Could you check a few things on this drawing? It's one solid part, dimensions in mm from its lowest x, y, z. A direction names the side the tool comes from. Round coordinates to 2 decimals unless told otherwise and drop trailing zeros. Loops run counter-clockwise (first coordinate to the right, second up) from the corner with the lowest first, then second, coordinate; pieces in that order, holes last. Notation, with made-up numbers: M 15.5,51 L 28.5,51 A17 cw 28.5,70 Z; hole C 7.5,-8 d10. An arc over 180 degrees is marked long. Put each result on its own line as item: value. Start each with the question number.
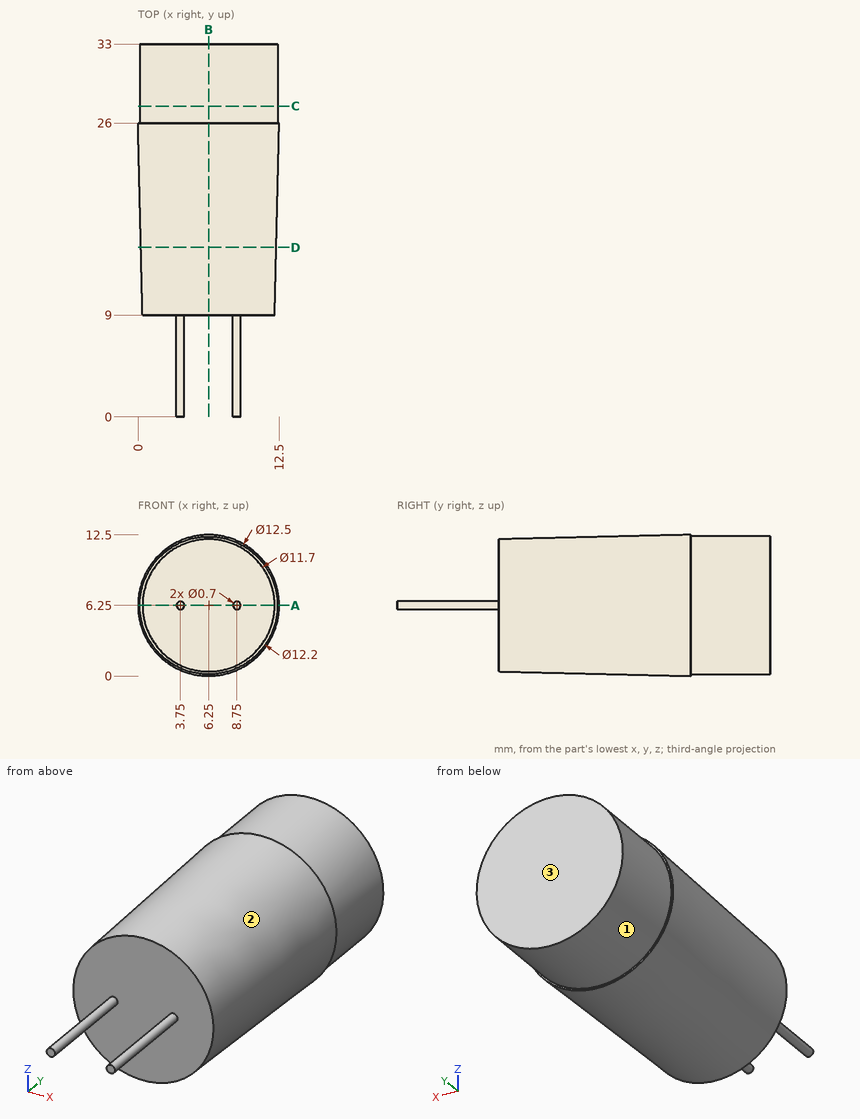
1) Suppose I cut it at B-B (x = 6.25). Write out the boundary of the cut face in (y, z).
2) I'm going to push flat-ended pins straight in: P1, Ø5, axis at y = 21, z = 1.5, coming from the -X side; P2, Ø3, axis at y = 7, z = 7.5, coming from the +X side; P3, Ø4, axis at x = 5, y = 23, coming from the -Z side. Where does each tip first touch, or does it pass through?
3) Suppose I cut it at D-D (y = 15). Write out the boundary of the cut face in (x, z), plus the area to 3 significant figures.
4) If I drill on probe 1 along Y at (x, z) = (2.75, 2.75); probe 2 along X at (y, z) = (28, 6.25); probe 3 along X at (y, z) = (4.5, 6), over which ranges is the centre line in solid material (lowest first)? Write a range as from..to.
5) Suppose I cut it at A-A (z = 6.25). Write out the boundary of the cut face in (x, y), plus the area to 3 significant figures.
6) On a 3-axis mill with a long thin cutter (end or side, diameter ignored), from which of +Z, -Z, +X, -X, +Y, -Y can I reach the whole of each face in a straight line? I mean the marked faces 1, 2 and 3. Say none if no direction works.
7) Suppose I cut it at C-C (y = 27.5). Write out the boundary of the cut face in (x, z).
Results are:
1. outline: M 9,0.4 L 26,0 L 26,0.15 L 33,0.15 L 33,12.35 L 26,12.35 L 26,12.5 L 9,12.1 Z
2. P1: x = 0.54
2. P2: x = 9.1
2. P3: z = 0.03
3. outline: C 6.25,6.25 d11.98
3. area: 113 mm²
4. probe 1: 9..33
4. probe 2: 0.15..12.35
4. probe 3: 3.51..3.99, 8.51..8.99
5. outline: M 0,26 L 0.4,9 L 3.4,9 L 3.4,0 L 4.1,0 L 4.1,9 L 8.4,9 L 8.4,0 L 9.1,0 L 9.1,9 L 12.1,9 L 12.5,26 L 12.35,26 L 12.35,33 L 0.15,33 L 0.15,26 Z
5. area: 304 mm²
6. face 1: +Y
6. face 2: -Y
6. face 3: +Z, -Z, +X, -X, +Y
7. outline: C 6.25,6.25 d12.2
